For this review, take the finished solid that the model builds, in its own axes (mm). Coordinates: 2 decimals unless noted, no trailing zeros. Loops run counter-clockwise (first coordinate to the right, second up) from the corner with the lowest first, then second, coordinate; pieces in that order, holes last.
1. Take a section at A-A, the plane z = 0.8. Count the separate pieces of the cut face and the enclosed holes in it, then the cut area to 3 significant figures.
2. To check wall thickness, follow probe 1 along Y at (x, z) = (-6, 1.1) (3 decimals); probe 2 along X at (y, z) = (15.5, 1.1); probe 3 along X at (y, z) = (11, 1.15). State the ranges of each line that lie inside material, in increasing order.
3. Take a section at B-B, the plane x = -9.5. State the section outline as (y, z) points (1 decimal).
4. Take a section at C-C, the plane y = 7.5. State the section outline as (x, z) points, then the cut area to 3 significant figures.
5. Clearance check with a flat-ended pin moving along its axis: P1, Ø0.9, axis at x = -19.46, y = -21.72, coming from the +Z side. State where the tip first meets the part, or that it passes through.
```python
from build123d import *

# Parameters (mm, degrees)
SKETCH1_R           = 0.6096
BOSS_EXTRUDE1_DEPTH = 1.5875


with BuildPart() as part:
    # Sketch1 → Boss-Extrude1 (new body)
    with BuildSketch(Plane.XY):
        with BuildLine():
            Line((30.48, -22.225), (29.415104476, -11.9888))
            ThreePointArc((29.415104476, -11.9888), (28.715873825, 1.490040556), (26.625688573, 14.824176893))
            ThreePointArc((26.625688573, 14.824176893), (23.941924767, 20.101731209), (18.415, 22.225))
            Line((18.415, 22.225), (-18.415, 22.225))
            ThreePointArc((-18.415, 22.225), (-23.941924767, 20.101731209), (-26.625688573, 14.824176893))
            ThreePointArc((-26.625688573, 14.824176893), (-28.715873825, 1.490040556), (-29.415104476, -11.9888))
            Line((-29.415104476, -11.9888), (-30.48, -22.225))
            Line((-30.48, -22.225), (-19.719346062, -22.225))
            ThreePointArc((-19.719346062, -22.225), (-19.457528855, -21.1455), (-19.195711648, -22.225))
            Line((-19.195711648, -22.225), (19.195711648, -22.225))
            ThreePointArc((19.195711648, -22.225), (19.457528855, -21.1455), (19.719346062, -22.225))
            Line((19.719346062, -22.225), (30.48, -22.225))
        make_face()
        with BuildLine():
            ThreePointArc((17.725268352, 19.939), (19.155271645, 17.728799653), (21.365471992, 19.158802947))
            ThreePointArc((21.365471992, 19.158802947), (23.441797038, 17.188737724), (24.362294321, 14.478577686))
            ThreePointArc((24.362294321, 14.478577686), (26.441646573, 1.258286409), (27.129050016, -12.106865432))
            Line((27.129050016, -12.106865432), (27.943845061, -19.939))
            Line((27.943845061, -19.939), (-27.943845061, -19.939))
            Line((-27.943845061, -19.939), (-27.129050016, -12.106865432))
            ThreePointArc((-27.129050016, -12.106865432), (-26.441646573, 1.258286409), (-24.362294321, 14.478577686))
            ThreePointArc((-24.362294321, 14.478577686), (-23.441797038, 17.188737724), (-21.365471992, 19.158802947))
            ThreePointArc((-21.365471992, 19.158802947), (-19.155271645, 17.728799653), (-17.725268352, 19.939))
            Line((-17.725268352, 19.939), (17.725268352, 19.939))
        make_face(mode=Mode.SUBTRACT)
        with Locations((19.457528855, 19.05)):
            Circle(SKETCH1_R, mode=Mode.SUBTRACT)
        with Locations((-19.457528855, 19.05)):
            Circle(SKETCH1_R, mode=Mode.SUBTRACT)
    extrude(amount=BOSS_EXTRUDE1_DEPTH)


solid = part.part
```
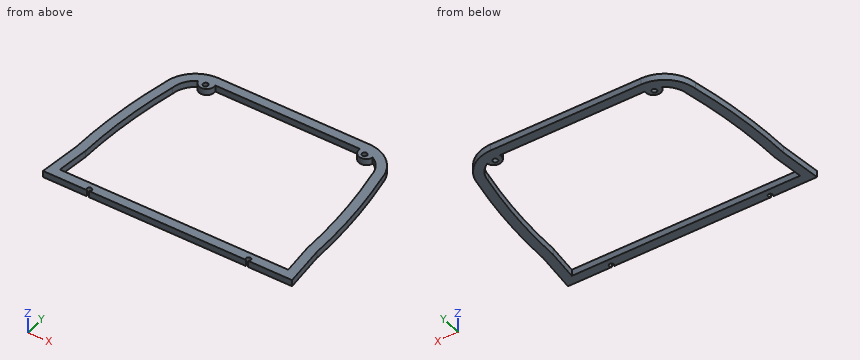
Results list:
1. separate pieces: 1
1. enclosed holes: 3
1. area: 438 mm2
2. probe 1: y = -22.225 to -19.939, 19.939 to 22.225
2. probe 2: x = -26.53 to -24.18, 24.18 to 26.53
2. probe 3: x = -27.37 to -25.05, 25.05 to 27.37
3. outline: (-22.2, 0) - (-19.9, 0) - (-19.9, 1.6) - (-22.2, 1.6) - close; (19.9, 0) - (22.2, 0) - (22.2, 1.6) - (19.9, 1.6) - close
4. outline: (-27.95, 0) - (-25.64, 0) - (-25.64, 1.59) - (-27.95, 1.59) - close; (25.64, 0) - (27.95, 0) - (27.95, 1.59) - (25.64, 1.59) - close
4. area: 7.34 mm2
5. P1: passes through
